Design review of the part built by this model. Coordinates are the model's own, in mm. A direction names the side the tool comes from. Coordinates: 2 decimals unless noted, no trailing zeros. Write each loop counter-clockwise with the first axis right and the second up, starting at its lowest first coordinate (ties: lowest second). Pieces come first, ordered by that corner, then holes. Notation, with made-up numbers: M 33.5,50.25 L 51.5,50.25 A17 cw 51.5,59.25 Z; hole C -0.75,2 d3. An arc over 180 degrees is marked long. One line per question, with ' | ' between items.
from build123d import *

# Parameters (mm, degrees)
SKETCH_1_W          = 58
SKETCH_1_H          = 25.4
EXTRUDE_1_DEPTH     = 3
SKETCH_2_W          = 8
SKETCH_2_H          = 3
EXTRUDE_2_DEPTH     = 28
SKETCH_3_R          = 3
CUT_EXTRUDE_1_DEPTH = 12
SKETCH_4_R          = 2
CUT_EXTRUDE_2_DEPTH = 22


with BuildPart() as part:
    # 草图1 → 凸台-拉伸1 (new body)
    with BuildSketch(Plane(origin=(0, 0, 0), x_dir=(1, 0, 0), z_dir=(0, 1, 0))):
        Rectangle(SKETCH_1_W, SKETCH_1_H)
    extrude(amount=EXTRUDE_1_DEPTH)

    # 草图2 → 凸台-拉伸2 (add)
    with BuildSketch(Plane(origin=(0, 3, 0), x_dir=(1, 0, 0), z_dir=(0, 1, 0))):
        with Locations((-24.75, 11.2)):
            Rectangle(SKETCH_2_W, SKETCH_2_H)
        with Locations((24.75, 11.2)):
            Rectangle(SKETCH_2_W, SKETCH_2_H)
        with Locations((-24.75, 0)):
            Rectangle(SKETCH_2_W, SKETCH_2_H)
        with Locations((24.75, 0)):
            Rectangle(SKETCH_2_W, SKETCH_2_H)
    extrude(amount=EXTRUDE_2_DEPTH)

    # 草图3 → 切除-拉伸1 (cut, symmetric)
    with BuildSketch(Plane.XY.offset(-9.7)):
        with Locations((-24.75, 12)):
            Circle(SKETCH_3_R)
        with Locations((-24.75, 22)):
            Circle(SKETCH_3_R)
        with Locations((24.75, 12)):
            Circle(SKETCH_3_R)
        with Locations((24.75, 22)):
            Circle(SKETCH_3_R)
    extrude(amount=CUT_EXTRUDE_1_DEPTH, both=True, mode=Mode.SUBTRACT)

    # 草图4 → 切除-拉伸2 (cut)
    with BuildSketch(Plane(origin=(0, 3, 0), x_dir=(1, 0, 0), z_dir=(0, 1, 0))):
        with Locations((24.75, -7.5)):
            Circle(SKETCH_4_R)
        with Locations((24.75, 7.5)):
            Circle(SKETCH_4_R)
        with Locations((-4.85, 7.5)):
            Circle(SKETCH_4_R)
        with Locations((-4.85, -7.5)):
            Circle(SKETCH_4_R)
    extrude(amount=-CUT_EXTRUDE_2_DEPTH, mode=Mode.SUBTRACT)


solid = part.part
1. Draft analysis for pull direction Z (two halves, no side actions). For faces 5 (the face through (-6.848, 1.521, 7.412)), 6 (the face through (-25, 17, 1.5)), 7 (the face through (-27.747, 22.132, -11.179)), state which applies: pulls with the +Z half, pulls with the -Z half, needs draft (parallel to the pull), parting line crosses it, or undercut.
Answer sheet:
face 5: undercut | face 6: pulls with the +Z half | face 7: needs draft
2. Insertion check: pin 1 Ø1.5 at (y, z) = (19.5, -0.5) entering from +X; pin 2 Ø4 at (y, z) = (16, 2) entering from -X; pin 3 Ø7 at (x, y) = (24.75, 22) entering from -Z; pin 4 Ø5 at (x, y) = (-24.75, 12) entering from -Z. Each pin has a flat end and moves straight along its axis. Give the tip position at first contact, or say it passes through.
Answer sheet:
pin 1: x = 28.75 | pin 2: x = -28.75 | pin 3: z = -12.7 | pin 4: through
3. Take a section at D-D (y = 6.5). Write out the cut boundary in (x, z).
Answer sheet:
outline: M -28.75,-12.7 L -20.75,-12.7 L -20.75,-9.7 L -28.75,-9.7 Z; M -28.75,-1.5 L -20.75,-1.5 L -20.75,1.5 L -28.75,1.5 Z; M 20.75,-12.7 L 28.75,-12.7 L 28.75,-9.7 L 20.75,-9.7 Z; M 20.75,-1.5 L 28.75,-1.5 L 28.75,1.5 L 20.75,1.5 Z
4. Take a section at A-A (y = 22). Count the separate pieces of the cut face and the enclosed holes in it, then the cut area to 3 significant figures.
Answer sheet:
separate pieces: 8 | enclosed holes: 0 | area: 24.0 mm^2
5. Tool access review of faces 1 (the face through (28.75, 17, -11)), 2 (the face through (-20.75, 17, -11)), 3 (the face through (25, 17, 1.5)), 4 (the face through (25, 17, -9.7)): name each direction out of +Z, -Z, +X, -X, +Y, -Y from which nothing blocks a thin tool from reaching the whole face with its end or side.
Answer sheet:
face 1: +Z, -Z, +X, +Y | face 2: +Z, -Z, +Y | face 3: +Z, +X, -X, +Y | face 4: +X, -X, +Y
6. To check wall thickness, follow line 1 along X through (y, z) = (1.15, 7.5); line 2 along Y through (x, z) = (-24.75, -0.9); line 3 along Z through (x, y) = (24.75, 2.2). State the ranges of each line that lie inside material, in increasing order. Write a range as [from, to].
Answer sheet:
line 1: [-29, -6.85], [-2.85, 22.75], [26.75, 29] | line 2: [0, 9], [15, 19], [25, 31] | line 3: [-12.7, -9.5], [-5.5, 5.5], [9.5, 12.7]
7. Take a section at B-B (z = -0.5). Write out the cut boundary in (x, y), then the cut area to 3 significant figures.
Answer sheet:
outline: M -29,0 L 29,0 L 29,3 L 28.75,3 L 28.75,31 L 20.75,31 L 20.75,3 L -20.75,3 L -20.75,31 L -28.75,31 L -28.75,3 L -29,3 Z; hole C -24.75,12 d6; hole C -24.75,22 d6; hole C 24.75,12 d6; hole C 24.75,22 d6 | area: 509 mm^2
